```python
from build123d import *

# Parameters (mm, degrees)
SKETCH2_R             = 1.5
BOSS_EXTRUDE2_DEPTH   = 3
BOSS_EXTRUDE2_2_DEPTH = 3
BOSS_EXTRUDE2_3_DEPTH = 3
BOSS_EXTRUDE2_4_DEPTH = 3
BOSS_EXTRUDE2_5_DEPTH = 3
BOSS_EXTRUDE2_6_DEPTH = 3
BOSS_EXTRUDE2_7_DEPTH = 3
BOSS_EXTRUDE2_8_DEPTH = 3
BOSS_EXTRUDE2_9_DEPTH = 3
SKETCH3_W             = 64.685996336
SKETCH3_H             = 8.346580173
CUT_EXTRUDE1_DEPTH    = 10


with BuildPart() as part:
    # Sketch2 → Boss-Extrude2 (new body)
    with BuildSketch(Plane(origin=(0, 0, 0), x_dir=(1, 0, 0), z_dir=(0, 1, 0))):
        with Locations(Location((24, 0, 0), (0, 0, 270))):
            Circle(SKETCH2_R)
    extrude(amount=BOSS_EXTRUDE2_DEPTH)


with BuildPart() as body_2:
    # Sketch2 → Boss-Extrude2 2 (new body)
    with BuildSketch(Plane(origin=(0, 0, 0), x_dir=(1, 0, 0), z_dir=(0, 1, 0))):
        with Locations(Location((32, 0, 0), (0, 0, 270))):
            Circle(SKETCH2_R)
    extrude(amount=BOSS_EXTRUDE2_2_DEPTH)


with BuildPart() as body_3:
    # Sketch2 → Boss-Extrude2 3 (new body)
    with BuildSketch(Plane(origin=(0, 0, 0), x_dir=(1, 0, 0), z_dir=(0, 1, 0))):
        with Locations(Location((40, 0, 0), (0, 0, 270))):
            Circle(SKETCH2_R)
    extrude(amount=BOSS_EXTRUDE2_3_DEPTH)


with BuildPart() as body_4:
    # Sketch2 → Boss-Extrude2 4 (new body)
    with BuildSketch(Plane(origin=(0, 0, 0), x_dir=(1, 0, 0), z_dir=(0, 1, 0))):
        with Locations(Location((48, 0, 0), (0, 0, 270))):
            Circle(SKETCH2_R)
    extrude(amount=BOSS_EXTRUDE2_4_DEPTH)


with BuildPart() as body_5:
    # Sketch2 → Boss-Extrude2 5 (new body)
    with BuildSketch(Plane(origin=(0, 0, 0), x_dir=(1, 0, 0), z_dir=(0, 1, 0))):
        with Locations(Location((56, 0, 0), (0, 0, 270))):
            Circle(SKETCH2_R)
    extrude(amount=BOSS_EXTRUDE2_5_DEPTH)


with BuildPart() as body_6:
    # Sketch2 → Boss-Extrude2 6 (new body)
    with BuildSketch(Plane(origin=(0, 0, 0), x_dir=(1, 0, 0), z_dir=(0, 1, 0))):
        with Locations(Location((64, 0, 0), (0, 0, 270))):
            Circle(SKETCH2_R)
    extrude(amount=BOSS_EXTRUDE2_6_DEPTH)


with BuildPart() as body_7:
    # Sketch2 → Boss-Extrude2 7 (new body)
    with BuildSketch(Plane(origin=(0, 0, 0), x_dir=(1, 0, 0), z_dir=(0, 1, 0))):
        with Locations(Location((72, 0, 0), (0, 0, 270))):
            Circle(SKETCH2_R)
    extrude(amount=BOSS_EXTRUDE2_7_DEPTH)


with BuildPart() as body_8:
    # Sketch2 → Boss-Extrude2 8 (new body)
    with BuildSketch(Plane(origin=(0, 0, 0), x_dir=(1, 0, 0), z_dir=(0, 1, 0))):
        with Locations(Location((80, 0, 0), (0, 0, 270))):
            Circle(SKETCH2_R)
    extrude(amount=BOSS_EXTRUDE2_8_DEPTH)


with BuildPart() as body_9:
    # Sketch2 → Boss-Extrude2 9 (new body)
    with BuildSketch(Plane(origin=(0, 0, 0), x_dir=(1, 0, 0), z_dir=(0, 1, 0))):
        with BuildLine():
            Line((0, 4), (16, 4))
            ThreePointArc((16, 4), (20, 0), (16, -4))
            Line((16, -4), (0, -4))
            ThreePointArc((0, -4), (-4, 0), (0, 4))
        make_face()
        with Locations(Location((0, 0, 0), (0, 0, 270))):
            Circle(SKETCH2_R, mode=Mode.SUBTRACT)
        with Locations(Location((8, 0, 0), (0, 0, 270))):
            Circle(SKETCH2_R, mode=Mode.SUBTRACT)
        with Locations(Location((16, 0, 0), (0, 0, 270))):
            Circle(SKETCH2_R, mode=Mode.SUBTRACT)
    extrude(amount=BOSS_EXTRUDE2_9_DEPTH)


with BuildPart() as cut_extrude1_tool:
    # Sketch3 → Cut-Extrude1 (new body)
    with BuildSketch(Plane.XZ):
        with Locations((54.20188262, -0.75152397)):
            Rectangle(SKETCH3_W, SKETCH3_H)
    extrude(amount=-CUT_EXTRUDE1_DEPTH)


with BuildPart() as part_1:
    add(part.part)

    # Cut-Extrude1: cut by cut_extrude1_tool
    add(cut_extrude1_tool.part, mode=Mode.SUBTRACT)


with BuildPart() as body_2_1:
    add(body_2.part)

    # Cut-Extrude1: cut by cut_extrude1_tool
    add(cut_extrude1_tool.part, mode=Mode.SUBTRACT)


with BuildPart() as body_3_1:
    add(body_3.part)

    # Cut-Extrude1: cut by cut_extrude1_tool
    add(cut_extrude1_tool.part, mode=Mode.SUBTRACT)


with BuildPart() as body_4_1:
    add(body_4.part)

    # Cut-Extrude1: cut by cut_extrude1_tool
    add(cut_extrude1_tool.part, mode=Mode.SUBTRACT)


with BuildPart() as body_5_1:
    add(body_5.part)

    # Cut-Extrude1: cut by cut_extrude1_tool
    add(cut_extrude1_tool.part, mode=Mode.SUBTRACT)


with BuildPart() as body_6_1:
    add(body_6.part)

    # Cut-Extrude1: cut by cut_extrude1_tool
    add(cut_extrude1_tool.part, mode=Mode.SUBTRACT)


with BuildPart() as body_7_1:
    add(body_7.part)

    # Cut-Extrude1: cut by cut_extrude1_tool
    add(cut_extrude1_tool.part, mode=Mode.SUBTRACT)


with BuildPart() as body_8_1:
    add(body_8.part)

    # Cut-Extrude1: cut by cut_extrude1_tool
    add(cut_extrude1_tool.part, mode=Mode.SUBTRACT)


solid = body_9.part
```
Part model, mm, in its own coordinate system. Round coordinates to 2 decimals unless told otherwise and drop trailing zeros. Write each loop counter-clockwise with the first axis right and the second up, starting at its lowest first coordinate (ties: lowest second). Pieces come first, ordered by that corner, then holes. Notation, with made-up numbers: M -2.75,63.5 L 19.25,63.5 A26 cw 19.25,92.5 Z; hole C 45.5,-1 d11. An arc over 180 degrees is marked long. Answer as CSV lines item,"result". Start each with the question number.
1) Drill centre lines: L1, parallel to X at y = 1.85, z = 0; L2, parallel to Z at x = -0.5, y = 0.2; L3, parallel to Z at x = 0.75, y = 2.25. Where is each one in solid material? Low to high.
2) Band-saw the part on B-B (y = 2.05). List the corners of the cut face in (x, z).
3) Band-saw the part on C-C (x = 8). List the corners of the cut face in (y, z), then the cut area to 3 significant figures.
4) Mould opens along X. For faces 1 (the face through (-4, 1, 0)), 2 (the face through (0.45, 1.48, 1.43)), 3 (the face through (8, 1, -4)), 4 (the face through (17.265, 1.479, 0.806)) say: +X half, -X half, draft (parallel to the pull), parting line (faces both ways), or undercut.
5) Band-saw the part on A-A (z = 0). List the corners of the cut face in (x, y).
6) Band-saw the part on D-D (z = -1.25). List the corners of the cut face in (x, y).
Worked out:
1,L1,"-4 to -1.5, 1.5 to 6.5, 9.5 to 14.5, 17.5 to 20"
1,L2,"-3.97 to -1.41, 1.41 to 3.97"
1,L3,"-4 to -1.3, 1.3 to 4"
2,outline,"M 0,-4 L 16,-4 A4 ccw 16,4 L 0,4 A4 ccw Z; hole C 0,0 d3; hole C 8,0 d3; hole C 16,0 d3"
3,outline,"M 0,-4 L 3,-4 L 3,-1.5 L 0,-1.5 Z; M 0,1.5 L 3,1.5 L 3,4 L 0,4 Z"
3,area,"15.0 mm²"
4,face 1,"-X half"
4,face 2,"undercut"
4,face 3,"draft"
4,face 4,"undercut"
5,outline,"M -4,0 L -1.5,0 L -1.5,3 L -4,3 Z; M 1.5,0 L 6.5,0 L 6.5,3 L 1.5,3 Z; M 9.5,0 L 14.5,0 L 14.5,3 L 9.5,3 Z; M 17.5,0 L 20,0 L 20,3 L 17.5,3 Z"
6,outline,"M -3.8,0 L -0.83,0 L -0.83,3 L -3.8,3 Z; M 0.83,0 L 7.17,0 L 7.17,3 L 0.83,3 Z; M 8.83,0 L 15.17,0 L 15.17,3 L 8.83,3 Z; M 16.83,0 L 19.8,0 L 19.8,3 L 16.83,3 Z"
